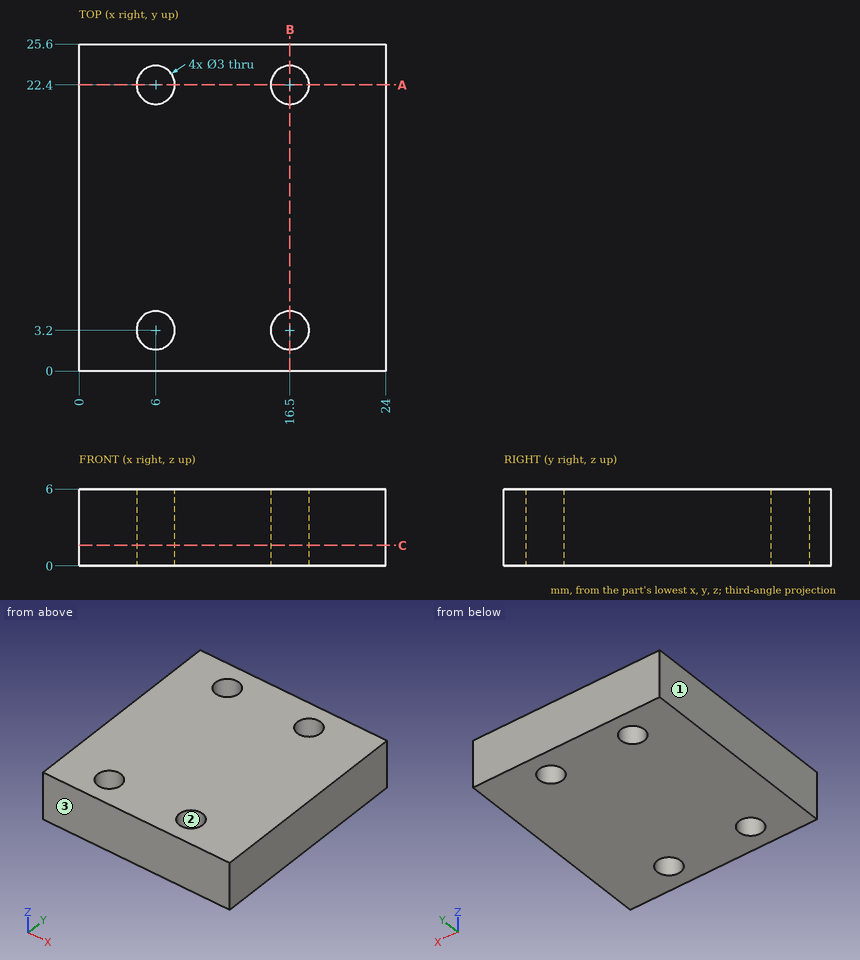
Source: three-view drawing plus pictorial views. Frame: mm from the lowest corner of the part. Coordinates: 2 decimals unless noted, no trailing zeros. Loops run counter-clockwise (first coordinate to the right, second up) from the corner with the lowest first, then second, coordinate; pieces in that order, holes last. Notation, with made-up numbers: (15.5, 89.25) -> (69.5, 89.25) arc R17 ccw to (69.5, 109.25) -> close; hole circle Ø7 at (-21, -7.75). An arc over 180 degrees is marked (long way). Write each question's results on one line, items separated by ' | '. Start each with the question number.
Q1. Pull-direction query (X, two-part tool) for the marked faces 1, 2 and 3; classes: released by +X, released by -X, zero draft, split by the parting line, or undercut.
Q2. Section A-A, the plane y = 22.4. Return the cut outline in (x, z).
Q3. Section C-C, the plane z = 1.6. Return the cut outline in (x, y), plus the area to 3 significant figures.
Q4. Pin query (flat end, axial travel): pin 1 (5 mm diameter, centred on x = 6, y = 3.2, fed in from -Z); pin 2 (2.5 mm diameter, centred on x = 16.5, y = 22.4, fed in from -Z). Return the tip coordinate at first contact, or that it passes through.
Q5. Ray query, line 1 (Y direction, x = 16.5, z = 2); line 2 (Y direction, x = 15.25, z = 3.9); line 3 (X direction, y = 21.5, z = 2.1). Return the intervals inside material, ascending. Write a range as from..to.
Q6. Section B-B, the plane x = 16.5. Return the cut outline in (y, z).
Found:
1) face 1: released by -X | face 2: undercut | face 3: zero draft
2) outline: (0, 0) -> (4.5, 0) -> (4.5, 6) -> (0, 6) -> close; (7.5, 0) -> (15, 0) -> (15, 6) -> (7.5, 6) -> close; (18, 0) -> (24, 0) -> (24, 6) -> (18, 6) -> close
3) outline: (0, 0) -> (24, 0) -> (24, 25.6) -> (0, 25.6) -> close; hole circle Ø3 at (6, 3.2); hole circle Ø3 at (6, 22.4); hole circle Ø3 at (16.5, 3.2); hole circle Ø3 at (16.5, 22.4) | area: 586 mm2
4) pin 1: z = 0 | pin 2: through
5) line 1: 0..1.7, 4.7..20.9, 23.9..25.6 | line 2: 0..2.37, 4.03..21.57, 23.23..25.6 | line 3: 0..4.8, 7.2..15.3, 17.7..24
6) outline: (0, 0) -> (1.7, 0) -> (1.7, 6) -> (0, 6) -> close; (4.7, 0) -> (20.9, 0) -> (20.9, 6) -> (4.7, 6) -> close; (23.9, 0) -> (25.6, 0) -> (25.6, 6) -> (23.9, 6) -> close
